Here's the drawing with two shaded views (mm, measured from the low corner). I have some questions. Coordinates: 2 decimals unless noted, no trailing zeros. Write each loop counter-clockwise with the first axis right and the second up, starting at its lowest first coordinate (ties: lowest second). Pieces come first, ordered by that corner, then holes. Notation, with made-up numbers: (52.25, -36) - (95.25, -36) arc R13 cw to (95.25, -16) - close; hole circle Ø11 at (-26.5, 32). An arc over 180 degrees is marked (long way). Answer in a Markdown table with one row per item. Add a question column.
Item 1: Imagine slicing it at B-B (x = 34). Please give me the cut outline in (y, z), plus the area to 3 significant figures.
Item 2: Imagine slicing it at D-D (x = 98.5). Please give me the cut outline in (y, z).
Item 3: If I drill on probe 1 along Z at (x, y) = (93, 1.3) (1 decimal); probe 2 along X at (y, z) = (0.4, 94) (1 decimal); probe 3 along Z at (x, y) = (65.5, 0.4), over which ranges is the centre line in solid material (lowest first)? Write a range as from..to.
Item 4: I'm going to push a flat-ended pin straight in: pin 1 (9 mm diameter, centred on x = 18.63, z = 76, fed in from +Y). Where does the tip first touch, or does it pass through?
Item 5: Imagine slicing it at A-A (z = 55). Please give me the cut outline in (x, y), plus the area to 3 significant figures.
Item 6: Imagine slicing it at C-C (z = 76). Please give me the cut outline in (x, y), plus the area to 3 significant figures.
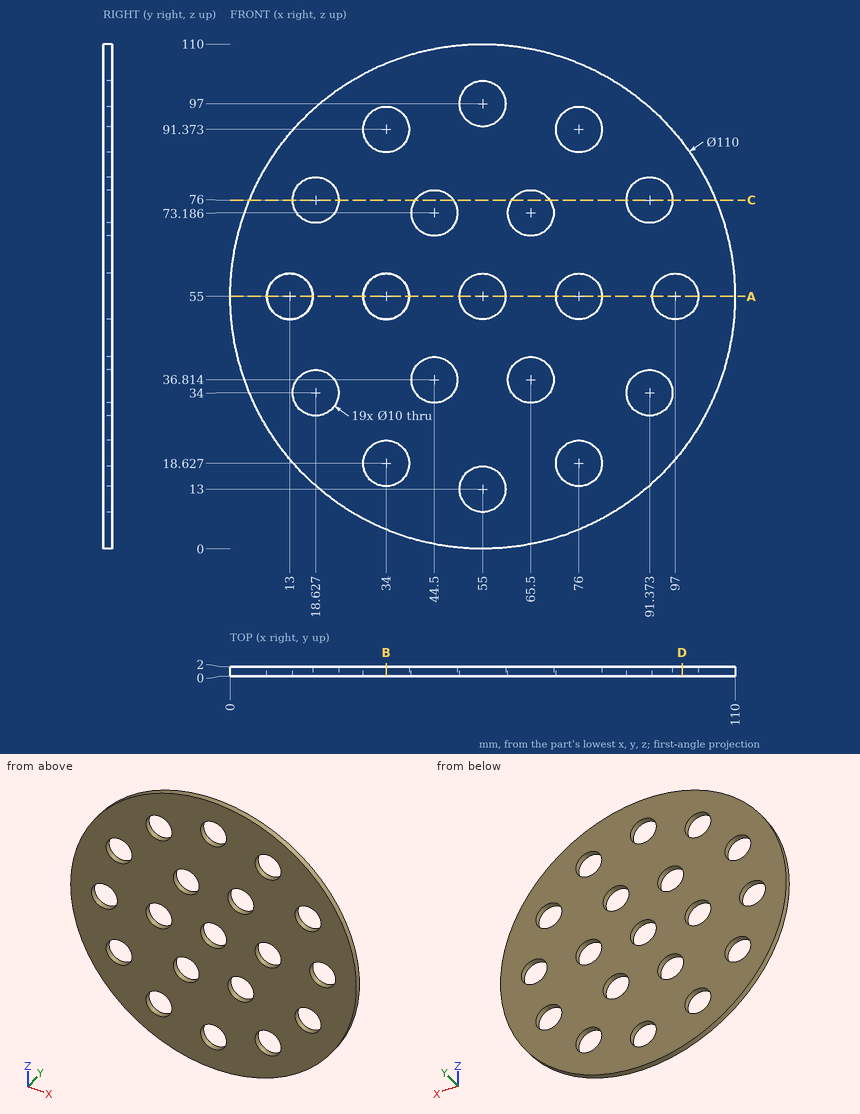
Here are the results:
| question | item | result |
|---|---|---|
| 1 | outline | (0, 4.17) - (2, 4.17) - (2, 13.63) - (0, 13.63) - close; (0, 23.63) - (2, 23.63) - (2, 50) - (0, 50) - close; (0, 60) - (2, 60) - (2, 86.37) - (0, 86.37) - close; (0, 96.37) - (2, 96.37) - (2, 105.83) - (0, 105.83) - close |
| 1 | area | 143 mm2 |
| 2 | outline | (0, 21.34) - (2, 21.34) - (2, 50.23) - (0, 50.23) - close; (0, 59.77) - (2, 59.77) - (2, 88.66) - (0, 88.66) - close |
| 3 | probe 1 | z = 15.2..29.3, 38.7..52, 58..71.3, 80.7..94.8 |
| 3 | probe 2 | x = 16.2..29.7, 38.3..51, 59..71.7, 80.3..93.8 |
| 3 | probe 3 | z = 1.01..31.81, 41.81..68.19, 78.19..108.99 |
| 4 | pin 1 | passes through |
| 5 | outline | (0, 0) - (8, 0) - (8, 2) - (0, 2) - close; (18, 0) - (29, 0) - (29, 2) - (18, 2) - close; (39, 0) - (50, 0) - (50, 2) - (39, 2) - close; (60, 0) - (71, 0) - (71, 2) - (60, 2) - close; (81, 0) - (92, 0) - (92, 2) - (81, 2) - close; (102, 0) - (110, 0) - (110, 2) - (102, 2) - close |
| 5 | area | 120 mm2 |
| 6 | outline | (4.17, 0) - (13.63, 0) - (13.63, 2) - (4.17, 2) - close; (23.63, 0) - (40.37, 0) - (40.37, 2) - (23.63, 2) - close; (48.63, 0) - (61.37, 0) - (61.37, 2) - (48.63, 2) - close; (69.63, 0) - (86.37, 0) - (86.37, 2) - (69.63, 2) - close; (96.37, 0) - (105.83, 0) - (105.83, 2) - (96.37, 2) - close |
| 6 | area | 130 mm2 |
